Autodesk Fusion 360 part; units mm, degrees
sketch "Sketch1" plane through (0, 0, 0) normal (0, 0, 1) x (1, 0, 0)
  line L0 (0, 0) -> (37, 0)
  line L1 (37, 0) -> (37, 49)
  line L2 (37, 49) -> (0, 49)
  line L3 (0, 49) -> (0, 0)
  line L4 (2, 2) -> (35, 2)
  line L5 (35, 2) -> (35, 47)
  line L6 (35, 47) -> (2, 47)
  line L7 (2, 47) -> (2, 2)
  circle A0 centre (4.5, 4.5) radius 0.8998
  circle A1 centre (32.5, 4.5) radius 0.9
  circle A2 centre (32.5, 44.5) radius 0.9002
  circle A3 centre (4.5, 44.5) radius 0.8999
  line L8 (3, 38) -> (34, 38)
  line L9 (34, 38) -> (34, 8)
  line L10 (34, 8) -> (3, 8)
  line L11 (3, 8) -> (3, 38)
  line L12 (2, 47) -> (7, 47)
  line L13 (7, 47) -> (7, 42)
  line L14 (7, 42) -> (2, 42)
  line L15 (2, 42) -> (2, 47)
  line L16 (35, 47) -> (30, 47)
  line L17 (30, 47) -> (30, 42)
  line L18 (30, 42) -> (35, 42)
  line L19 (35, 42) -> (35, 47)
  line L20 (35, 2) -> (30, 2)
  line L21 (30, 2) -> (30, 7)
  line L22 (30, 7) -> (35, 7)
  line L23 (35, 7) -> (35, 2)
  line L24 (2, 2) -> (7, 2)
  line L25 (7, 2) -> (7, 7)
  line L26 (7, 7) -> (2, 7)
  line L27 (2, 7) -> (2, 2)
extrude "Extrude1" add sketch "Sketch1" along normal blind 1 contours L0 L1 L2 L3 | L4 L7 L24 L25 L26 L27 | L4 L5 L6 L7 L13 L14 L17 L18 L21 L22 L25 L26 | L4 L5 L20 L21 L22 L23 | L6 L7 L12 L13 L14 L15 | L5 L6 L16 L17 L18 L19 | A0 | A1 | A2 | A3
extrude "Extrude2" cut sketch "Sketch1" along normal blind 4 contours L4 L7 L24 L25 L26 L27 | L4 L5 L20 L21 L22 L23 | L6 L7 L12 L13 L14 L15 | L5 L6 L16 L17 L18 L19 | A0 | A1 | A2 | A3
extrude "Extrude3" add sketch "Sketch1" along normal blind 4 contours L4 L7 L24 L25 L26 L27 | L4 L5 L20 L21 L22 L23 | L6 L7 L12 L13 L14 L15 | L5 L6 L16 L17 L18 L19 | A0 | A1 | A2 | A3
extrude "Extrude4" cut sketch "Sketch1" along normal blind 5 contours A0 | A1 | A2 | A3
extrude "Extrude5" add sketch "Sketch1" along normal blind 6 contours A0 | A1 | A2 | A3
extrude "Extrude6" cut sketch "Sketch1" along normal blind 4 contours L0 L1 L2 L3
extrude "Extrude7" add sketch "Sketch1" along normal blind 6 contours L0 L1 L2 L3
extrude "Extrude8" cut 4 faces at (4.5224, 2.5343, 4) (32.5224, 2.5342, 4) (4.5224, 42.5342, 4) (32.4776, 42.5341, 4) along direction (0, 0, -1) blind 1
extrude "Extrude9" cut 5 faces at (32.5668, 44.2075, 6) (0.6667, 17, 6) (4.65, 44.2402, 6) (4.7199, 4.7934, 6) (32.7134, 4.9094, 6) along direction (0, 0, -1) blind 1
Source: CAD feature listing. Evaluate the final solid. Frame: model axes, mm. A direction names the side the tool comes from. Round coordinates to 2 decimals unless told otherwise and drop trailing zeros. Loops run counter-clockwise (first coordinate to the right, second up) from the corner with the lowest first, then second, coordinate; pieces in that order, holes last.
1. Section query D-D on z = 1.7. Output: boundary loops of the cut face in (x, y), and give its area (3 significant figures).
2. Section query A-A on z = 3.9. Output: boundary loops of the cut face in (x, y).
3. Section query C-C on x = 32.5. Output: boundary loops of the cut face in (y, z).
4. Section query B-B on y = 15.5. Output: boundary loops of the cut face in (x, z), and give its area (3 significant figures).
5. Ray query, L1, parallel to X at y = 46, z = 2.65; L2, parallel to Y at x = 16, z = 2.7; L3, parallel to X at y = 31.5, z = 1.3. Return the intervals inside material, ascending.
6. Mould query, pull axis Y, two halves, no side actions, for faces 1 (the flat face through (37, 24, 2)), 2 (the flat face through (31, 45, 3)), 3 (the flat face through (19, 49, 2)), 4 (the flat face through (34, 23.2, 0.5)). Classes: released by +Y, released by -Y, zero draft, split by the parting line, or undercut.
7. Access query for faces 5 (the flat face through (35, 24, 3)), 6 (the flat face through (32, 5, 5)). Directions: +Z, -Z, +X, -X, +Y, -Y. A direction counts if a zero-diameter tool reaches every point of the face in a straight line with its end or side. Return the directions, or none.
Answers below:
1. outline: (0, 0) - (37, 0) - (37, 49) - (0, 49) - close; hole (2, 7) - (7, 7) - (7, 2) - (30, 2) - (30, 7) - (35, 7) - (35, 42) - (30, 42) - (30, 47) - (7, 47) - (7, 42) - (2, 42) - close
1. area: 428 mm2
2. outline: (0, 0) - (37, 0) - (37, 49) - (0, 49) - close; circle Ø1.8 at (4.5, 4.5); circle Ø1.8 at (4.5, 44.5); circle Ø1.8 at (32.5, 4.5); circle Ø1.8 at (32.5, 44.5); hole (2, 2) - (35, 2) - (35, 47) - (2, 47) - close
3. outline: (0, 0) - (8, 0) - (8, 1) - (7, 1) - (7, 3) - (5.4, 3) - (5.4, 5) - (3.6, 5) - (3.6, 3) - (2, 3) - (2, 5) - (0, 5) - close; (38, 0) - (49, 0) - (49, 5) - (47, 5) - (47, 3) - (45.4, 3) - (45.4, 5) - (43.6, 5) - (43.6, 3) - (42, 3) - (42, 1) - (38, 1) - close
4. outline: (0, 0) - (3, 0) - (3, 1) - (2, 1) - (2, 5) - (0, 5) - close; (34, 0) - (37, 0) - (37, 5) - (35, 5) - (35, 1) - (34, 1) - close
4. area: 22.0 mm2
5. L1: x = 0 to 7, 30 to 37
5. L2: y = 0 to 2, 47 to 49
5. L3: x = 0 to 2, 35 to 37
6. face 1: zero draft
6. face 2: undercut
6. face 3: released by +Y
6. face 4: undercut
7. face 5: +Z
7. face 6: +Z, +X, -X, +Y, -Y
